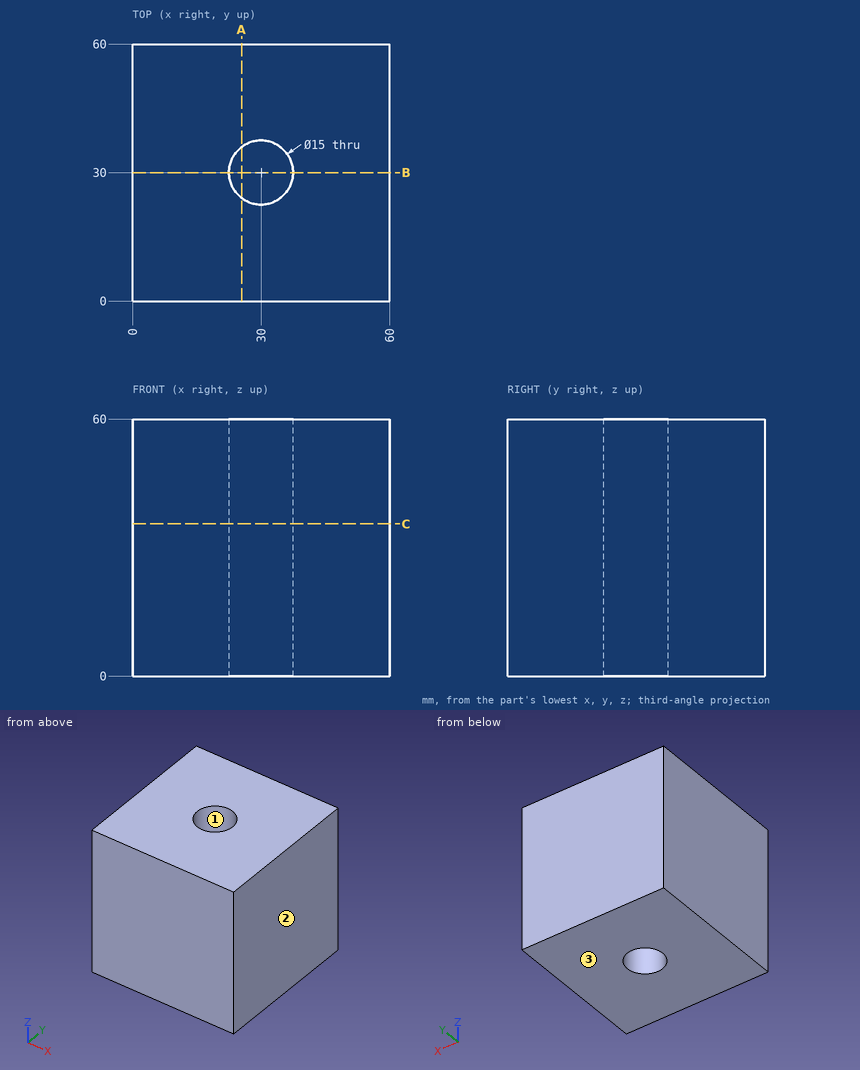
Could you check a few things on this drawing? It's one solid part, dimensions in mm from its lowest x, y, z. Coordinates: 2 decimals unless noted, no trailing zeros. Loops run counter-clockwise (first coordinate to the right, second up) from the corner with the lowest first, then second, coordinate; pieces in that order, holes last. Notation, with made-up numbers: (62.25, 54) - (66.25, 54) arc R11 ccw to (66.25, 75) - close; hole circle Ø1 at (5.5, 54). An arc over 180 degrees is marked (long way). Answer as a JSON object with one key per item and string values. Group by question number.
Item 1: If I drill on L1, parallel to X at y = 30, z = 41.5; L2, parallel to Y at x = 34, z = 21.5, over which ranges is the centre line in solid material (lowest first)? Write a range as from..to.
Item 2: If we mould it in two halves opening along X, with no side actions, what happens to the marked faces 1, 2 and 3? For each: released by +X, released by -X, zero draft, split by the parting line, or undercut.
Item 3: If we section it at C-C (z = 35.5): List the corners of the cut face in (x, y) for me, plus the area to 3 significant figures.
Item 4: If we section it at B-B (y = 30): List the corners of the cut face in (x, z) for me.
Item 5: If we section it at A-A (x = 25.5): List the corners of the cut face in (y, z) for me.
Returned:
{
 "1": {"L1": "x = 0..22.5, 37.5..60", "L2": "y = 0..23.66, 36.34..60"},
 "2": {"face 1": "undercut", "face 2": "released by +X", "face 3": "zero draft"},
 "3": {"outline": "(0, 0) - (60, 0) - (60, 60) - (0, 60) - close; hole circle Ø15 at (30, 30)", "area": "3,420 mm²"},
 "4": {"outline": "(0, 0) - (22.5, 0) - (22.5, 60) - (0, 60) - close; (37.5, 0) - (60, 0) - (60, 60) - (37.5, 60) - close"},
 "5": {"outline": "(0, 0) - (24, 0) - (24, 60) - (0, 60) - close; (36, 0) - (60, 0) - (60, 60) - (36, 60) - close"}
}
